from build123d import *

# Parameters (mm, degrees)
SKETCH007_W       = 12.5
SKETCH007_H       = 12
PAD004_DEPTH      = 15
PAD004_DEPTH_BACK = 3
FILLET006_R       = 3
SKETCH008_W       = 6.9
SKETCH008_H       = 9.4
POCKET005_DEPTH   = 22
SKETCH009_R       = 1.75
POCKET006_DEPTH   = 12
CHAMFER005_SIZE   = 1
CHAMFER006_SIZE   = 0.2
CHAMFER007_SIZE   = 2
POCKET007_DEPTH   = 2


with BuildPart() as but_e:
    # Sketch007 → Pad004 (new body, two sides)
    with BuildSketch(Plane.YZ) as pad004_sk:
        Rectangle(SKETCH007_W, SKETCH007_H)
    extrude(amount=PAD004_DEPTH)
    extrude(pad004_sk.sketch, amount=-PAD004_DEPTH_BACK)

    # Fillet006
    fillet006_edges = [but_e.edges().sort_by_distance(p)[0] for p in [
        (-3, 0, 6),
        (-3, 0, -6),
    ]]
    fillet(fillet006_edges, radius=FILLET006_R)

    # Sketch008 → Pocket005 (cut)
    with BuildSketch(Plane.YZ):
        Rectangle(SKETCH008_W, SKETCH008_H)
    extrude(amount=POCKET005_DEPTH, mode=Mode.SUBTRACT)

    # Sketch009 → Pocket006 (cut, symmetric)
    with BuildSketch(Plane.XZ):
        with Locations((9, 0)):
            Circle(SKETCH009_R)
    extrude(amount=POCKET006_DEPTH, both=True, mode=Mode.SUBTRACT)

    # Chamfer005
    chamfer005_edges = [but_e.edges().sort_by_distance(p)[0] for p in [
        (7.5, -6.25, 6),
        (7.5, 6.25, 6),
    ]]
    chamfer(chamfer005_edges, length=CHAMFER005_SIZE)

    # Chamfer006
    chamfer006_edges = [but_e.edges().sort_by_distance(p)[0] for p in [
        (15, -6.25, 0),
        (15, -5.75, -5.5),
        (15, -5.75, 5.5),
        (15, 0, -6),
        (15, 0, 6),
        (15, 5.75, -5.5),
        (15, 5.75, 5.5),
        (15, 6.25, 0),
        (15, -3.45, 0),
        (15, 0, -4.7),
        (15, 3.45, 0),
        (15, 0, 4.7),
        (7.25, -3.45, 0),
        (7.25, 3.45, 0),
    ]]
    chamfer(chamfer006_edges, length=CHAMFER006_SIZE)

    # Chamfer007
    chamfer007_edges = [but_e.edges().sort_by_distance(p)[0] for p in [
        (7.25, 6.25, 0),
    ]]
    chamfer(chamfer007_edges, length=CHAMFER007_SIZE)

    # Sketch010 (on Face34 of Chamfer007) → Pocket007 (cut)
    with BuildSketch(Plane.XZ.offset(6.25)):
        Polygon((12.204294, 0), (10.602147, 2.775), (7.397853, 2.775), (5.795706, 0), (7.397853, -2.775), (10.602147, -2.775), align=None)
    extrude(amount=-POCKET007_DEPTH, mode=Mode.SUBTRACT)


with BuildPart() as but_e_1:
    # Body003 placement: moved
    add(but_e.part.moved(Location((-75, 3.25, 0))))


with BuildPart() as part_mirroring001:
    add(but_e_1.part.mirror(Plane(origin=(0, 0, 0), x_dir=(0, -1, 0), z_dir=(1, 0, 0))))


solid = part_mirroring001.part
Work out the finished part from the listing and answer in its coordinate system (mm). A direction names the side the tool comes from. Give positions to 0.01 mm unless a question says otherwise; leave off trailing zeros. Order: outer loops, then holes, each group sorted by start corner. A loop starts at its lowest first (then second) coordinate and runs counter-clockwise, first axis right, second up. Notation, with made-up numbers: (-24.75, 56.25) -> (-6.75, 56.25) arc R22 cw to (-6.75, 65.25) -> close; hole circle Ø5 at (61, 36.5). An arc over 180 degrees is marked (long way). One line per item, written item: value.
Item 1: Find section A-A, the plane y = -0.75. Give the vertices of the cut face in (x, z).
Answer sheet:
outline: (60, -5.8) -> (60.2, -6) -> (75, -6) arc R3 ccw to (78, -3) -> (78, 3) arc R3 ccw to (75, 6) -> (60.2, 6) -> (60, 5.8) -> close; hole circle Ø3.5 at (66, 0)
Item 2: Find section D-D, the plane y = 7.75. Give the vertices of the cut face in (x, z), plus the area to 3 significant figures.
Answer sheet:
outline: (60, -5.8) -> (60.2, -6) -> (75, -6) arc R3 ccw to (78, -3) -> (78, 3) arc R3 ccw to (75, 6) -> (60.2, 6) -> (60, 5.8) -> close; hole circle Ø4 at (66, 0)
area: 200 mm²
Item 3: Straight lines are drawn through the part: probe 1 along Z at (x, y) = (66, 7.2); probe 2 along Y at (x, z) = (61.25, 3.5); probe 3 along X at (y, z) = (-2.5, -0.5). For each, find the intervals that lie inside material, in ascending order.
Answer sheet:
probe 1: -6 to -1.75, 1.75 to 6
probe 2: -3 to -0.2, 6.7 to 9.5
probe 3: 60 to 63.08, 68.92 to 77.5
Item 4: Determine the mould class of faces 1 (the flat face through (67.7, 9, -5.5)), 2 (the flat face through (66, -2, 2.775)), 3 (the flat face through (77.5, -2.5, 0)) for opening direction X: released by +X, released by -X, zero draft, split by the parting line, or undercut.
Answer sheet:
face 1: zero draft
face 2: undercut
face 3: released by +X
Item 5: Flat-ended cylindrical pins translate along their axes: P1, Ø5.5, axis at x = 66, z = 0, coming from the +Y side; P2, Ø3, axis at x = 66, z = -1, coming from the +Y side; P3, Ø1.7, axis at x = 67, z = -1, coming from the -Y side. Find the tip coordinate at first contact, or state that the pin passes through.
Answer sheet:
P1: y = 8.5
P2: y = 8.25
P3: y = -1
Item 6: A tool of negligible diameter and unlimited length cuts with its end or side. For faces 4 (the flat face through (75, 3, 0)), 5 (the flat face through (63.586, -2.014, 1.368)), 6 (the flat face through (67, 3, 6)), from which of +Z, -Z, +X, -X, +Y, -Y can it reach the whole face along a straight path? Write none if from no direction.
Answer sheet:
face 4: -X
face 5: -Y
face 6: +Z, +X, -X, +Y, -Y
Item 7: Find section C-C, the plane x = 72.5. Give the vertices of the cut face in (y, z).
Answer sheet:
outline: (-3, -5) -> (-2, -6) -> (8.5, -6) -> (9.5, -5) -> (9.5, 5) -> (8.5, 6) -> (-2, 6) -> (-3, 5) -> close; hole (-0.2, -4.7) -> (6.7, -4.7) -> (6.7, 4.7) -> (-0.2, 4.7) -> close
